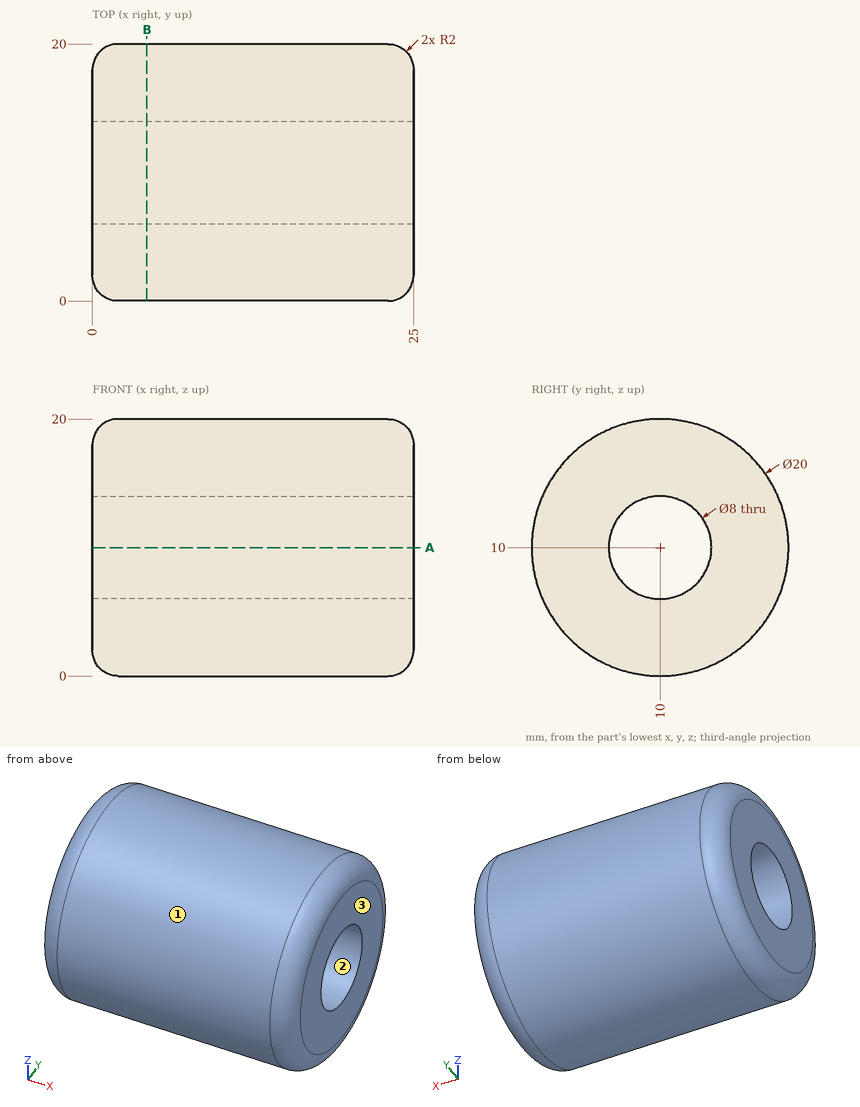
Answer from the drawing. Dimensions are ordinates in mm from the lowest x, y and z of the part. Give positions to 0.01 mm unless a question says otherwise; leave off trailing zeros. Order: outer loops, then holes, each group sorted by start corner. A loop starts at its lowest first (then second) coordinate and runs counter-clockwise, first axis right, second up. Notation, with made-up numbers: (-39, 86) - (6, 86) arc R10 ccw to (6, 99) - close; hole circle Ø8 at (-32, 63.25). An arc over 180 degrees is marked (long way). One line per item, written item: value. Start each with the question number.
1. Section A-A, the plane z = 10 is taken. Write down the section's boundary in (x, y), then the cut area to 3 significant figures.
2. Consider line 1 (Y direction, x = 16.5, z = 10); line 2 (Y direction, x = 10.75, z = 16); line 3 (Y direction, x = 10.75, z = 9.25). Determine where each line is inside the solid, lowest interval first.
3. Section B-B, the plane x = 4.25 is taken. Write down the section's boundary in (y, z), then the cut area to 3 significant figures.
4. For a pull along Y with two mould halves and no side action, classify the marked faces 1, 2 and 3 as released by +Y, released by -Y, zero draft, split by the parting line, or undercut.
5. Each of these flat-tipped pins is pushed along its axis until it touches: pin 1 Ø2 at (x, z) = (22, 15.5) entering from +Y; pin 2 Ø5 at (y, z) = (10, 10) entering from +X; pin 3 Ø5 at (x, y) = (20.5, 8.5) entering from -Z; pin 4 Ø1 at (x, y) = (17.5, 6.5) entering from -Z. Where does it stop, or does it pass through?
Filled sheet:
1. outline: (0, 2) arc R2 ccw to (2, 0) - (23, 0) arc R2 ccw to (25, 2) - (25, 6) - (0, 6) - close; (0, 14) - (25, 14) - (25, 18) arc R2 ccw to (23, 20) - (2, 20) arc R2 ccw to (0, 18) - close
1. area: 297 mm²
2. line 1: 0 to 6, 14 to 20
2. line 2: 2 to 18
2. line 3: 0.03 to 6.07, 13.93 to 19.97
3. outline: circle Ø20 at (10, 10); hole circle Ø8 at (10, 10)
3. area: 264 mm²
4. face 1: split by the parting line
4. face 2: undercut
4. face 3: zero draft
5. pin 1: y = 18.93
5. pin 2: through
5. pin 3: z = 0
5. pin 4: z = 0.46
